Work out the finished part from the listing and answer in its coordinate system (mm). A direction names the side the tool comes from. Give positions to 0.01 mm unless a question says otherwise; leave off trailing zeros. Use CSV: the item, a comma, the result in double quotes.
from build123d import *
from OCP.BRepFilletAPI import BRepFilletAPI_MakeChamfer

# Parameters (mm, degrees)
ESQUISSE1_W             = 100
ESQUISSE1_H             = 100
BOSS_EXTRU_1_DEPTH      = 3
ESQUISSE2_W             = 65.1
ESQUISSE2_H             = 16.1
ENL_V_MAT_EXTRU_1_DEPTH = 142.453172464
CHANFREIN1_SIZE         = 3
ESQUISSE3_W             = 5
ESQUISSE3_H             = 5
ESQUISSE3_R             = 1.3
BOSS_EXTRU_2_DEPTH      = 7.85
CHANFREIN2_SIZE         = 1.732050808
CHANFREIN2_SIZE_2       = 3
CONG_1_R                = 1
ESQUISSE4_W             = 10
ESQUISSE4_H             = 5
BOSS_EXTRU_3_DEPTH      = 10
ESQUISSE5_R             = 1.7
ENL_V_MAT_EXTRU_2_DEPTH = 10


with BuildPart() as part:
    # Esquisse1 → Boss.-Extru.1 (new body)
    with BuildSketch(Plane.XY):
        with Locations((50, 50)):
            Rectangle(ESQUISSE1_W, ESQUISSE1_H)
    extrude(amount=BOSS_EXTRU_1_DEPTH)

    # Esquisse2 → Enlèv. mat.-Extru.1 (cut, through all)
    with BuildSketch(Plane.XY.offset(3)):
        with Locations((50, 76.95)):
            Rectangle(ESQUISSE2_W, ESQUISSE2_H)
    extrude(amount=-ENL_V_MAT_EXTRU_1_DEPTH, mode=Mode.SUBTRACT)

    # Chanfrein1
    chanfrein1_edges = [part.edges().sort_by_distance(p)[0] for p in [
        (50, 0, 3),
        (0, 50, 3),
        (50, 100, 3),
        (100, 50, 3),
    ]]
    chamfer(chanfrein1_edges, length=CHANFREIN1_SIZE - 0.0001)  # a hair under: the kernel refuses the full size

    # Esquisse3 → Boss.-Extru.2 (add)
    # profile 1 of 4: a face of its own
    with BuildSketch(Plane(origin=(0, 0, 0), x_dir=(-1, 0, 0), z_dir=(0, 0, -1))):
        with Locations((-87.5, 92.45)):
            Rectangle(ESQUISSE3_W, ESQUISSE3_H)
        with Locations((-87.5, 92.45)):
            Circle(ESQUISSE3_R, mode=Mode.SUBTRACT)
    # profile 2 of 4: a face of its own
    with BuildSketch(Plane(origin=(0, 0, 0), x_dir=(-1, 0, 0), z_dir=(0, 0, -1))):
        with Locations((-12.5, 92.45)):
            Rectangle(ESQUISSE3_W, ESQUISSE3_H)
        with Locations((-12.5, 92.45)):
            Circle(ESQUISSE3_R, mode=Mode.SUBTRACT)
    # profile 3 of 4: a face of its own
    with BuildSketch(Plane(origin=(0, 0, 0), x_dir=(-1, 0, 0), z_dir=(0, 0, -1))):
        with Locations((-87.5, 61.45)):
            Rectangle(ESQUISSE3_W, ESQUISSE3_H)
        with Locations((-87.5, 61.45)):
            Circle(ESQUISSE3_R, mode=Mode.SUBTRACT)
    # profile 4 of 4: a face of its own
    with BuildSketch(Plane(origin=(0, 0, 0), x_dir=(-1, 0, 0), z_dir=(0, 0, -1))):
        with Locations((-12.5, 61.45)):
            Rectangle(ESQUISSE3_W, ESQUISSE3_H)
        with Locations((-12.5, 61.45)):
            Circle(ESQUISSE3_R, mode=Mode.SUBTRACT)
    extrude(amount=BOSS_EXTRU_2_DEPTH)

    # Chanfrein2
    chanfrein2_edges_1 = [part.edges().sort_by_distance(p)[0] for p in [
        (82.55, 76.95, 3),
    ]]
    chanfrein2_side_1 = [part.faces().sort_by_distance(p)[0] for p in [
        (82.584641016, 76.95, 3),
    ]]
    chanfrein2_edges_2 = [part.edges().sort_by_distance(p)[0] for p in [
        (50, 68.9, 3),
    ]]
    chanfrein2_side_2 = [part.faces().sort_by_distance(p)[0] for p in [
        (50, 68.865358984, 3),
    ]]
    chanfrein2_edges_3 = [part.edges().sort_by_distance(p)[0] for p in [
        (17.45, 76.95, 3),
    ]]
    chanfrein2_side_3 = [part.faces().sort_by_distance(p)[0] for p in [
        (17.415358984, 76.95, 3),
    ]]
    chanfrein2_edges_4 = [part.edges().sort_by_distance(p)[0] for p in [
        (50, 85, 3),
    ]]
    chanfrein2_side_4 = [part.faces().sort_by_distance(p)[0] for p in [
        (50, 85.034641016, 3),
    ]]
    chanfrein2 = BRepFilletAPI_MakeChamfer(part.part.solid().wrapped)
    for e in chanfrein2_edges_1:
        chanfrein2.Add(CHANFREIN2_SIZE - 0.0001, CHANFREIN2_SIZE_2 - 0.0001, e.wrapped, chanfrein2_side_1[0].wrapped)
    for e in chanfrein2_edges_2:
        chanfrein2.Add(CHANFREIN2_SIZE - 0.0001, CHANFREIN2_SIZE_2 - 0.0001, e.wrapped, chanfrein2_side_2[0].wrapped)
    for e in chanfrein2_edges_3:
        chanfrein2.Add(CHANFREIN2_SIZE - 0.0001, CHANFREIN2_SIZE_2 - 0.0001, e.wrapped, chanfrein2_side_3[0].wrapped)
    for e in chanfrein2_edges_4:
        chanfrein2.Add(CHANFREIN2_SIZE - 0.0001, CHANFREIN2_SIZE_2 - 0.0001, e.wrapped, chanfrein2_side_4[0].wrapped)
    add(Compound.cast(chanfrein2.Shape()), mode=Mode.REPLACE)  # a hair under: the kernel refuses the full size

    # Congé1
    cong_1_edges = [part.edges().sort_by_distance(p)[0] for p in [
        (90, 92.45, 0),
        (87.5, 89.95, 0),
        (85, 92.45, 0),
        (87.5, 94.95, 0),
        (15, 92.45, 0),
        (12.5, 89.95, 0),
        (10, 92.45, 0),
        (12.5, 94.95, 0),
        (90, 61.45, 0),
        (87.5, 58.95, 0),
        (85, 61.45, 0),
        (87.5, 63.95, 0),
        (15, 61.45, 0),
        (12.5, 58.95, 0),
        (10, 61.45, 0),
        (12.5, 63.95, 0),
    ]]
    fillet(cong_1_edges, radius=CONG_1_R)

    # Esquisse4 → Boss.-Extru.3 (add)
    with BuildSketch(Plane(origin=(0, 0, 0), x_dir=(-1, 0, 0), z_dir=(0, 0, -1))):
        with Locations((-94.95, 37.5)):
            Rectangle(ESQUISSE4_W, ESQUISSE4_H)
        with Locations((-5.05, 37.5)):
            Rectangle(ESQUISSE4_W, ESQUISSE4_H)
    extrude(amount=BOSS_EXTRU_3_DEPTH)

    # Esquisse5 → Enlèv. mat.-Extru.2 (cut)
    with BuildSketch(Plane.XZ.offset(-35)):
        with Locations(Location((94.95, -5.05, 0), (0, 0, 270))):
            Circle(ESQUISSE5_R)
        with Locations(Location((5.05, -5.05, 0), (0, 0, 270))):
            Circle(ESQUISSE5_R)
    extrude(amount=-ENL_V_MAT_EXTRU_2_DEPTH, mode=Mode.SUBTRACT)


solid = part.part
Item 1: For faces 1 (the flat face through (83.404, 76.813, 1.479)), 2 (the flat face through (88, 63.95, -4)), 3 (the cylindrical face through (86.3, 91.95, -3.87)), 4 (the flat face through (85, 61, -4)), 5 (the flat face through (13, 94.95, -4)), determine the directions among +Z, -Z, +X, -X, +Y, -Y from which every point of the face is accessible in a straight line to the end or side of a thin tool.
Determined:
face 1,"+Z"
face 2,"-Z, +X, -X"
face 3,"-Z"
face 4,"-Z, +Y, -Y"
face 5,"-Z, +X, -X, +Y"
Item 2: Find the intervals of material crossed by line 1 (X direction, y = 38.3, z = -5.05); line 2 (Y direction, x = 12.5, z = -3); line 3 (X direction, y = 62, z = -2.75), in increasing order.
Determined:
line 1,"x = 0.05 to 3.35, 6.75 to 10.05, 89.95 to 93.25, 96.65 to 99.95"
line 2,"y = 58.95 to 60.15, 62.75 to 63.95, 89.95 to 91.15, 93.75 to 94.95"
line 3,"x = 10 to 11.32, 13.68 to 15, 85 to 86.32, 88.68 to 90"
Item 3: The mould has two halves that part along Z. Classify faces 6 (the cylindrical face through (93.29, 37.47, -4.68)), 7 (the flat face through (90, 61, -4)), 8 (the cylindrical face through (4.4, 37.47, -6.62)), 9 (the flat face through (87, 61, 0)): pulls with the +Z half, pulls with the -Z half, needs draft (parallel to the pull), parting line crosses it, or undercut.
Determined:
face 6,"undercut"
face 7,"needs draft"
face 8,"undercut"
face 9,"pulls with the -Z half"
Item 4: A cutting plane is placed at C-C on z = -5.05. State how many separate pieces and enclosed holes the cut face has, and give its area (3 significant figures).
Determined:
separate pieces,"8"
enclosed holes,"4"
area,"145 mm²"
Item 5: Given P1, Ø3, axis at x = 4.5, z = -5.5, coming from the +Y side; P2, Ø2.5, axis at x = 12, z = -4, coming from the +Y side; P3, Ø10, axis at x = 76, y = 12, coming from the -Z side, each flat-ended and moving along its own axis, determine where each tip first touches the part or whether it passes through.
Determined:
P1,"stops at y = 40"
P2,"stops at y = 94.95"
P3,"stops at z = 0"
